```python
from build123d import *

# Parameters (mm, degrees)
CUT_EXTRUDE1_DEPTH       = 156.00175185
CUT_EXTRUDE1_DEPTH_BACK  = 156.00175185
SKETCH2_R                = 16
BOSS_EXTRUDE1_REACH      = 167.413
BOSS_EXTRUDE1_END_RADIUS = 45.5
SKETCH4_R                = 19
SKETCH4_R_2              = 16
CUT_EXTRUDE2_DEPTH       = 156.001751924
CUT_EXTRUDE2_DEPTH_BACK  = 156.001751924


with BuildPart() as part:
    # Sketch1 → Revolve1 (revolve)
    with BuildSketch(Plane(origin=(0, 0, 0), x_dir=(1, 0, 0), z_dir=(0, 1, 0)), mode=Mode.PRIVATE) as revolve1_sk:
        with BuildLine():
            Line((0, 131.958489975), (0, 116.958489975))
            ThreePointArc((0, 116.958489975), (23.090251563, 114.969167301), (45.5, 109.059827497))
            Line((45.5, 109.059827497), (45.5, 0))
            Line((45.5, 0), (57.5, 0))
            Line((57.5, 0), (57.5, 85))
            Line((57.5, 85), (53.5, 85))
            Line((53.5, 85), (53.5, 88))
            Line((53.5, 88), (57.5, 88))
            Line((57.5, 88), (57.5, 90.5))
            Line((57.5, 90.5), (53.5, 90.5))
            Line((53.5, 90.5), (53.5, 93.5))
            Line((53.5, 93.5), (57.5, 93.5))
            Line((57.5, 93.5), (57.5, 96))
            Line((57.5, 96), (53.5, 96))
            Line((53.5, 96), (53.5, 99))
            Line((53.5, 99), (57.5, 99))
            Line((57.5, 99), (57.5, 101.5))
            Line((57.5, 101.5), (53.5, 101.5))
            Line((53.5, 101.5), (53.5, 104.5))
            Line((53.5, 104.5), (57.5, 104.5))
            Line((57.5, 104.5), (57.5, 120.5))
            ThreePointArc((57.5, 120.5), (29.315298875, 129.065978744), (0, 131.958489975))
        make_face()
    revolve(revolve1_sk.sketch.rotate(Axis((0, 0, -138.64598988), (0, 0, 1)), 180), axis=Axis((0, 0, -138.64598988), (0, 0, 1)))

    # Sketch2 → Cut-Extrude1 (cut, two sides: drawn at the far end of the back side and taken through both)
    with BuildSketch(Plane(origin=(0, 0, 0), x_dir=(1, 0, 0), z_dir=(0, 1, 0)).offset(-CUT_EXTRUDE1_DEPTH_BACK)):
        with Locations(Location((0, 45, 0), (0, 0, 270))):
            Circle(SKETCH2_R)
    extrude(amount=CUT_EXTRUDE1_DEPTH + CUT_EXTRUDE1_DEPTH_BACK, mode=Mode.SUBTRACT)

    # Boss-Extrude1: up to this cylinder (the profile starts inside it)
    boss_extrude1_end = Plane(origin=(0, 0, -26.537401), z_dir=(0, 0, -1)) * Cylinder(BOSS_EXTRUDE1_END_RADIUS, 426.826, mode=Mode.PRIVATE)
    # Sketch4 → Boss-Extrude1 (add, up to the surface)
    with BuildSketch(Plane(origin=(0, 24, 0), x_dir=(1, 0, 0), z_dir=(0, 1, 0)), mode=Mode.PRIVATE) as boss_extrude1_sk1:
        with Locations(Location((0, 45, 0), (0, 0, 90))):
            Circle(SKETCH4_R)
        with Locations(Location((0, 45, 0), (0, 0, 270))):
            Circle(SKETCH4_R_2, mode=Mode.SUBTRACT)
    boss_extrude1_tool1 = extrude(boss_extrude1_sk1.sketch, amount=BOSS_EXTRUDE1_REACH, mode=Mode.PRIVATE) & boss_extrude1_end
    boss_extrude1 = boss_extrude1_tool1.solids().sort_by_distance((0, 24, -26.537401))[0]
    add(boss_extrude1)

    # Mirror1: Boss-Extrude1 across plane
    add(boss_extrude1.mirror(Plane.ZX))

    # Sketch5 → Cut-Extrude2 (cut, two sides: drawn at the far end of the back side and taken through both)
    with BuildSketch(Plane(origin=(0, 0, 0), x_dir=(1, 0, 0), z_dir=(0, 1, 0)).offset(-CUT_EXTRUDE2_DEPTH_BACK)):
        with BuildLine():
            Line((-30, 0), (30, 0))
            ThreePointArc((30, 0), (0, 15), (-30, 0))
        make_face()
    extrude(amount=CUT_EXTRUDE2_DEPTH + CUT_EXTRUDE2_DEPTH_BACK, mode=Mode.SUBTRACT)


solid = part.part
```
Work out the finished part from the listing and answer in its coordinate system (mm). A direction names the side the tool comes from. Give positions to 0.01 mm unless a question says otherwise; leave off trailing zeros. Write each loop counter-clockwise with the first axis right and the second up, starting at its lowest first coordinate (ties: lowest second). Pieces come first, ordered by that corner, then holes.
(1) Flat-ended cylindrical pins translate along their axes: pin 1 Ø1.5 at (x, y) = (10.5, -14) entering from +Z; pin 2 Ø19 at (x, z) = (-9.5, -47.5) entering from -Y; pin 3 Ø12 at (x, z) = (-21.5, -104) entering from -Y; pin 4 Ø19 at (x, z) = (0, -45) entering from +Y. Find the tip coordinate at first contact, or state that the pin passes through.
Final values:
pin 1: stops at z = -115.72
pin 2: stops at y = -56.5
pin 3: stops at y = -55.37
pin 4: passes through
(2) Straight lines are drawn through the part: line 1 (X direction, y = 37, z = -45); line 2 (Z direction, x = 3, y = -40.5); line 3 (Z direction, x = 0, y = 53.75). For each, find the intervals that lie inside material, in ascending order.
Final values:
line 1: x = -44.01 to -26.48, -19 to -16, 16 to 19, 26.48 to 44.01
line 2: z = -126.36 to -110.71, -63.76 to -60.72, -29.28 to -26.24
line 3: z = -122 to -104.5, -101.5 to -99, -96 to -93.5, -90.5 to -88, -85 to -61, -29 to -15
(3) The part is cut by section B-B on x = 0. Count the separate pieces of the cut face and the enclosed holes in it, plus the area to 3 significant figures.
Final values:
separate pieces: 3
enclosed holes: 0
area: 3,370 mm2
(4) The part is cut by section A-A on z = -34. Write down the section's boundary in (x, y), plus the area to 3 significant figures.
Final values:
outline: (-15.49, -42.78) arc R45.5 cw to (-15.49, 42.78) - (-15.49, 24) - (-11.62, 24) - (-11.62, 56.31) arc R57.5 ccw to (-11.62, -56.31) - (-11.62, -24) - (-15.49, -24) - close; (11.62, -56.31) arc R57.5 ccw to (11.62, 56.31) - (11.62, 24) - (15.49, 24) - (15.49, 42.78) arc R45.5 cw to (15.49, -42.78) - (15.49, -24) - (11.62, -24) - close
area: 3,620 mm2
(5) The mould has two halves that part along Z. Classify faces 4 (the cylindrical face through (12.465, 56.133, -89.268)), 5 (the cylindrical face through (42.46, 32.55, -97.52)), 6 (the cylindrical face through (0, 48, -15)): pulls with the +Z half, pulls with the -Z half, needs draft (parallel to the pull), parting line crosses it, or undercut.
Final values:
face 4: needs draft
face 5: undercut
face 6: pulls with the +Z half
(6) Which of the six approach directions +Z, -Z, +X, -X, +Y, -Y give full straight-line access (tool end or side, diameter ignored) to faces 1 (the flat face through (-17, 51, -101.5)), 2 (the flat face through (47, -1, 0)), 3 (the flat face through (13, -24, -35))?
Final values:
face 1: none
face 2: +Z, +X, -X, +Y, -Y
face 3: +Z
(7) The part is cut by section D-D on z = -111. Write down the section's boundary in (x, y).
Final values:
outline: circle Ø115 at (0, 0); hole circle Ø79.33 at (0, 0)
